The figure shows three views and two pictorial views of one solid part (mm, origin at its lowest corner). Answer the questions. Round coordinates to 2 decimals unless told otherwise and drop trailing zeros. Order: outer loops, then holes, each group sorted by start corner. A loop starts at its lowest first (then second) coordinate and runs counter-clockwise, first axis right, second up. Notation, with made-up numbers: (12, -9.5) - (45, -9.5) arc R21 cw to (45, 5.5) - close; hole circle Ø5 at (-11.75, 80.5). An arc over 180 degrees is marked (long way). Answer in a Markdown table with one row per item.
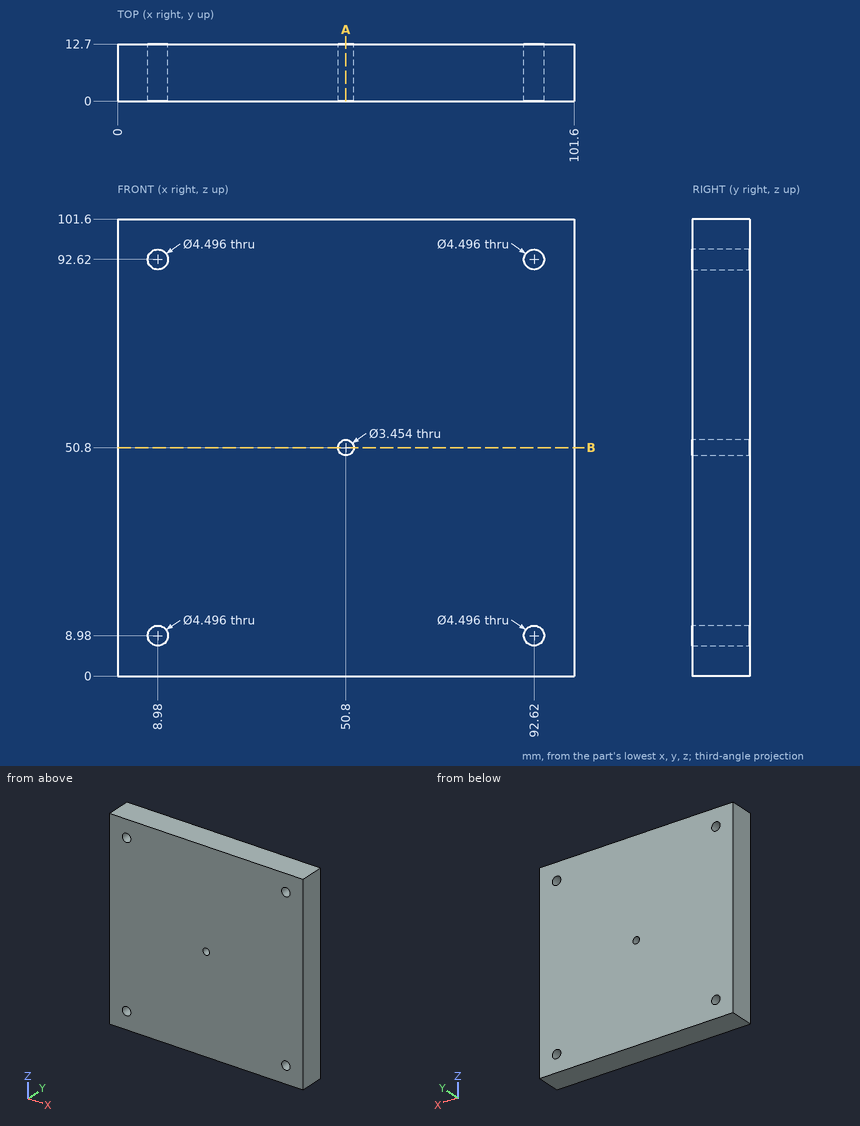
1) Find section A-A, the plane x = 50.8. Give the vertices of the cut face in (y, z).
Filled in:
| item | result |
|---|---|
| outline | (0, 0) - (12.7, 0) - (12.7, 49.07) - (0, 49.07) - close; (0, 52.53) - (12.7, 52.53) - (12.7, 101.6) - (0, 101.6) - close |
2) Find the intervals of material crossed by probe 1 along X at (y, z) = (7.75, 92); probe 2 along X at (y, z) = (7.25, 50.8); probe 3 along Z at (x, y) = (7, 1) (1 decimal), in increasing order. Write a range as from..to.
Filled in:
| item | result |
|---|---|
| probe 1 | x = 0..6.82, 11.14..90.46, 94.78..101.6 |
| probe 2 | x = 0..49.07, 52.53..101.6 |
| probe 3 | z = 0..7.9, 10..91.6, 93.7..101.6 |
3) This flat-tipped pin is pushed along its axis until it touches: pin 1 (4 mm diameter, centred on x = 92.62, z = 8.98, fed in from +Y). Where does it stop, or does it pass through?
Filled in:
| item | result |
|---|---|
| pin 1 | passes through |
4) Find section B-B, the plane z = 50.8. Give the vertices of the cut face in (x, y), then the cut area to 3 significant figures.
Filled in:
| item | result |
|---|---|
| outline | (0, 0) - (49.07, 0) - (49.07, 12.7) - (0, 12.7) - close; (52.53, 0) - (101.6, 0) - (101.6, 12.7) - (52.53, 12.7) - close |
| area | 1,250 mm^2 |
